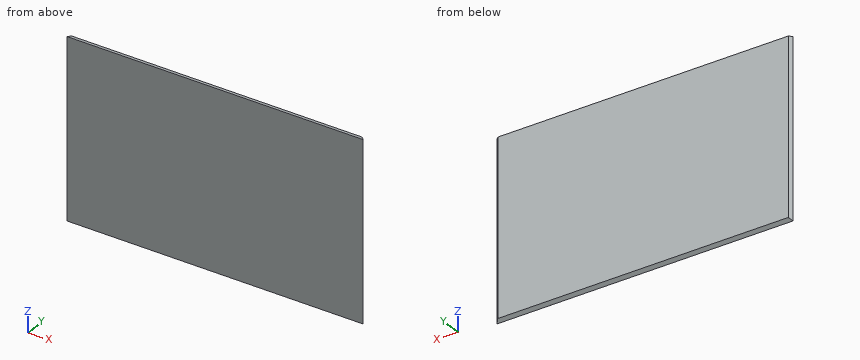
Autodesk Inventor part; units mm, degrees
ref_plane "YZ Plane" through (0, 0, 0) normal (1, 0, 0) x (0, 1, 0)
ref_plane "XZ Plane" through (0, 0, 0) normal (0, 1, 0) x (-1, 0, 0)
ref_plane "XY Plane" through (0, 0, 0) normal (0, 0, 1) x (1, 0, 0)
sketch "Skizze1" plane through (0, 0, 0) normal (0, 0, 1) x (1, 0, 0)
  line L0 (153.5, 0) -> (152, 1.5)
  line L1 (0, 0) -> (153.5, 0)
  line L2 (152, 1.5) -> (1.5, 1.5)
  line L3 (1.5, 1.5) -> (0, 0)
  dimension "d0" = 45
extrude "Extrusion1" add sketch "Skizze1" against normal blind 93
chamfer "Fase1" distance 1.5 angle 45 1 edges at (76.75, 1.5, -93)
properties part number "Zwischenplatt"
The model under review builds one solid part; all positions refer to its coordinate system, in mm. Round coordinates to 2 decimals unless told otherwise and drop trailing zeros. Loops run counter-clockwise (first coordinate to the right, second up) from the corner with the lowest first, then second, coordinate; pieces in that order, holes last. Notation, with made-up numbers: M 42.5,48.25 L 73.5,48.25 A22 ccw 73.5,77.25 Z; hole C -26,75 d6. An arc over 180 degrees is marked long. Answer as a JSON object with one key per item and string values.
Item 1: Clearance check with a flat-ended pin moving along its axis: P1, Ø1, axis at x = 72, z = -74.5, coming from the -Y side. State where the tip first meets the part, or that it passes through.
Check sheet entries:
{"P1": "y = 0"}
Item 2: We need section A-A, the plane y = 0.7. State the section outline as (x, z) points.
Check sheet entries:
{"outline": "M 0.7,-92.3 L 152.8,-92.3 L 152.8,0 L 0.7,0 Z"}
Item 3: For line 1 along Z through (x, y) = (68.5, 1.35); line 2 along Z through (x, y) = (126, 0.8); line 3 along X through (y, z) = (0.95, -38.5), list the stretches that pass through material, from the lowest coordinate up.
Check sheet entries:
{"line 1": "-91.65 to 0", "line 2": "-92.2 to 0", "line 3": "0.95 to 152.55"}
